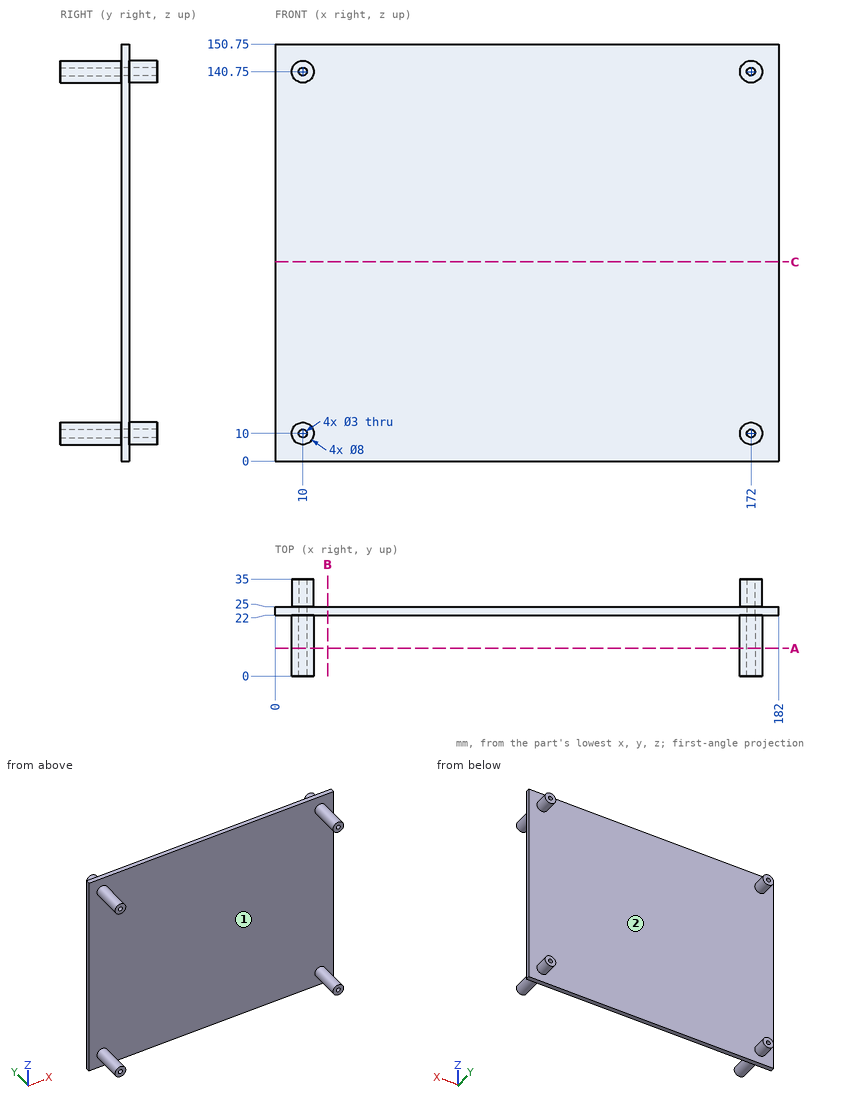
Study the drawing (mm; zero at the part's minimum x, y, z) and answer. A direction names the side the tool comes from. Coordinates: 2 decimals unless noted, no trailing zeros. Loops run counter-clockwise (first coordinate to the right, second up) from the corner with the lowest first, then second, coordinate; pieces in that order, holes last. Notation, with made-up numbers: (-35.5, -15) -> (11.5, -15) arc R6 ccw to (11.5, -10) -> close; hole circle Ø5 at (9, 79). An arc over 180 degrees is marked (long way). Answer in a Markdown table with one row per item. Add a question column.
1. Flat-ended cylindrical pins translate along their axes: P1, Ø12, axis at x = 151.5, z = 59, coming from the -Y side; P2, Ø8, axis at x = 127, z = 63, coming from the +Y side. Find the tip coordinate at first contact, or state that the pin passes through.
2. The part is cut by section B-B, the plane x = 19. Write down the section's boundary in (y, z).
3. For the marked faces 1 and 2, determine the directions among +Z, -Z, +X, -X, +Y, -Y from which every point of the face is accessible in a straight line to the end or side of a thin tool.
4. Consider line 1 (Z direction, x = 10, y = 31); line 2 (Z direction, x = 9.5, y = 13) (1 decimal); line 3 (X direction, y = 8, z = 10). Determine where each line is inside the solid, lowest interval first. Write a range as [from, to].
5. The part is cut by section A-A, the plane y = 10. Write down the section's boundary in (x, z).
6. The part is cut by section C-C, the plane z = 72. Write down the section's boundary in (x, y), then the cut area to 3 significant figures.
Answer below:
| question | item | result |
|---|---|---|
| 1 | P1 | y = 22 |
| 1 | P2 | y = 25 |
| 2 | outline | (22, 0) -> (25, 0) -> (25, 150.75) -> (22, 150.75) -> close |
| 3 | face 1 | -Y |
| 3 | face 2 | +Y |
| 4 | line 1 | [6, 8.5], [11.5, 14], [136.75, 139.25], [142.25, 144.75] |
| 4 | line 2 | [6, 8.6], [11.4, 14], [136.8, 139.3], [142.2, 144.7] |
| 4 | line 3 | [6, 8.5], [11.5, 14], [168, 170.5], [173.5, 176] |
| 5 | outline | circle Ø8 at (10, 10); circle Ø8 at (10, 140.75); circle Ø8 at (172, 10); circle Ø8 at (172, 140.75); hole circle Ø3 at (10, 10); hole circle Ø3 at (10, 140.75); hole circle Ø3 at (172, 10); hole circle Ø3 at (172, 140.75) |
| 6 | outline | (0, 22) -> (182, 22) -> (182, 25) -> (0, 25) -> close |
| 6 | area | 546 mm2 |
